```python
from build123d import *

# Parameters (mm, degrees)
F0_R     = 9.525
F0_W     = 19.05
F0_H     = 76.2
F0_W_2   = 19.048609
F1_DEPTH = 19.05


with BuildPart() as f1:
    # F0 (on Top) → F1 (new body)
    with BuildSketch(Plane.XY):
        Polygon((-287.56197, 204.938772), (-287.56197, -201.461228), (17.23803, -201.461228), (322.03803, -201.461228), (322.03803, 204.938772), (322.03803, 865.338772), (322.03803, 941.538772), (322.03803, 1068.538772), (626.83803, 1068.538772), (626.83803, 1627.338772), (525.23803, 1627.338772), (525.23803, 1170.138772), (449.03803, 1170.138772), (449.03803, 1627.338772), (-414.56197, 1627.338772), (-414.56197, 1170.138772), (-490.76197, 1170.138772), (-490.76197, 1627.338772), (-592.36197, 1627.338772), (-592.36197, 1068.538772), (-287.56197, 1068.538772), (-287.56197, 941.538772), (-287.56197, 865.338772), (-287.56197, 763.738772), (-287.56197, 687.538772), (-287.56197, 560.538772), align=None)
        with Locations((17.23803, 1.738772)):
            Circle(F0_R, mode=Mode.SUBTRACT)
        with Locations((-258.98697, 725.638772)):
            Rectangle(F0_W, F0_H, mode=Mode.SUBTRACT)
        with Locations((-258.98697, 903.438772)):
            Rectangle(F0_W, F0_H, mode=Mode.SUBTRACT)
        with Locations((291.380524, 724.869366)):
            Rectangle(F0_W, F0_H, mode=Mode.SUBTRACT)
        with Locations((293.463726, 903.438772)):
            Rectangle(F0_W_2, F0_H, mode=Mode.SUBTRACT)
    extrude(amount=F1_DEPTH)


solid = f1.part
```
Read the model definition and answer for the solid it produces. Units are mm, in the model's axes. Round coordinates to 2 decimals unless told otherwise and drop trailing zeros. Write each loop counter-clockwise with the first axis right and the second up, starting at its lowest first coordinate (ties: lowest second). Pieces come first, ordered by that corner, then holes. Notation, with made-up numbers: (29.25, -33) -> (77.25, -33) arc R32 cw to (77.25, -5) -> close; hole circle Ø2 at (-11.75, 78.25). An arc over 180 degrees is marked (long way). Answer in a Markdown table with one row per item. Add a question column.
1) Find section B-B, the plane z = 9.25. State how many separate pieces and enclosed holes the cut face has, and give its area (3 significant figures).
2) Find section A-A, the plane y = 1400. Determine the outline of the cut face in (x, z), and give its area (3 significant figures).
3) Find section D-D, the plane y = 742. Determine the outline of the cut face in (x, z).
4) Given P1, Ø1.5, axis at y = 580, z = 2.5, coming from the +X side; P2, Ø5.5, axis at x = 483, z = 11, coming from the +Y side; P3, Ø15, axis at x = 17.24, y = 1.74, coming from the +Z side; P4, Ø6, axis at x = 379.5, z = 10, coming from the -Y side, each flat-ended and moving along its own axis, determine where each tip first touches the part or whether it passes through.
5) Consider line 1 (X direction, y = 1272, z = 4); line 2 (Y direction, x = 297, z = 18); line 3 (X direction, y = 899, z = 14.5). Determine where each line is inside the solid, lowest interval first.
6) Find section C-C, the plane x = -317.5. Determine the outline of the cut face in (y, z).
Findings below:
| question | item | result |
|---|---|---|
| 1 | separate pieces | 1 |
| 1 | enclosed holes | 5 |
| 1 | area | 1,380,000 mm² |
| 2 | outline | (-592.36, 0) -> (-490.76, 0) -> (-490.76, 19.05) -> (-592.36, 19.05) -> close; (-414.56, 0) -> (449.04, 0) -> (449.04, 19.05) -> (-414.56, 19.05) -> close; (525.24, 0) -> (626.84, 0) -> (626.84, 19.05) -> (525.24, 19.05) -> close |
| 2 | area | 20,300 mm² |
| 3 | outline | (-287.56, 0) -> (-268.51, 0) -> (-268.51, 19.05) -> (-287.56, 19.05) -> close; (-249.46, 0) -> (281.86, 0) -> (281.86, 19.05) -> (-249.46, 19.05) -> close; (300.91, 0) -> (322.04, 0) -> (322.04, 19.05) -> (300.91, 19.05) -> close |
| 4 | P1 | x = 322.04 |
| 4 | P2 | y = 1170.14 |
| 4 | P3 | through |
| 4 | P4 | y = 1068.54 |
| 5 | line 1 | -592.36 to -490.76, -414.56 to 449.04, 525.24 to 626.84 |
| 5 | line 2 | -201.46 to 686.77, 762.97 to 865.34, 941.54 to 1627.34 |
| 5 | line 3 | -287.56 to -268.51, -249.46 to 283.94, 302.99 to 322.04 |
| 6 | outline | (1068.54, 0) -> (1627.34, 0) -> (1627.34, 19.05) -> (1068.54, 19.05) -> close |
